Verification items for the finished model (mm, model axes). Face numbers are marked on the shaded views. A direction names the side the tool comes from. Give positions to 0.01 mm unless a question says otherwise; leave off trailing zeros. Loops run counter-clockwise (first coordinate to the right, second up) from the corner with the lowest first, then second, coordinate; pieces in that order, holes last. Notation, with made-up numbers: M 8.5,25 L 15.5,25 A16 ccw 15.5,34 Z; hole C -39.75,2.5 d4. An arc over 180 degrees is marked long. Use CSV: the item, a comma, the result in double quotes.
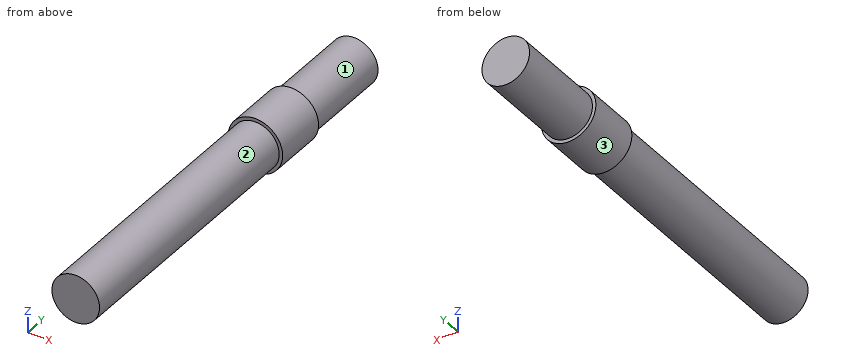
from build123d import *

# Parameters (mm, degrees)
F0_R      = 22.225
F1_DEPTH  = 406.4
F3_R      = 25.4
F4_DEPTH  = 50.8
F1_FACE_R = 22.225
F5_DEPTH  = 12.7


with BuildPart() as f1:
    # F0 (on Front) → F1 (new body)
    with BuildSketch(Plane.XZ):
        Circle(F0_R)
    extrude(amount=F1_DEPTH)

    # F3 (on offset) → F4 (join)
    with BuildSketch(Plane.XZ.offset(152.4)):
        Circle(F3_R)
    extrude(amount=-F4_DEPTH)

    # F1_face (on face) → F5 (cut)
    with BuildSketch(Plane(origin=(0, 0, 0), x_dir=(1, 0, 0), z_dir=(0, 1, 0))):
        Circle(F1_FACE_R)
    extrude(amount=-F5_DEPTH, mode=Mode.SUBTRACT)


solid = f1.part
(1) Depth check by flat-ended pin: pin 1 Ø4 at (y, z) = (-237.5, -2) entering from +X (3 decimals); pin 2 Ø1 at (x, y) = (-13.5, -360) entering from -Z; pin 3 Ø2 at (x, y) = (-11.5, -158) entering from +Z. Enter the tip coordinate at first touch or a pass-through.
Calculated:
pin 1,"stops at x = 22.225"
pin 2,"stops at z = -18.03"
pin 3,"stops at z = 19.59"
(2) Section check C-C on y = -169. Record the cut outline in (x, z) (3 decimals).
Calculated:
outline,"C 0,0 d44.45"
(3) Scan lines: L1, parallel to Y at x = 16.5, z = -17.5; L2, parallel to X at y = -370, z = 1.5; L3, parallel to Z at x = -19.5, y = -247. Record each from-to range of solid material in increasing order. Write a range as from..to.
Calculated:
L1,"y = -152.4..-101.6"
L2,"x = -22.17..22.17"
L3,"z = -10.66..10.66"
(4) Section check A-A on x = 0. Record the cut outline in (y, z) (3 decimals).
Calculated:
outline,"M -406.4,-22.225 L -152.4,-22.225 L -152.4,-25.4 L -101.6,-25.4 L -101.6,-22.225 L -12.7,-22.225 L -12.7,22.225 L -101.6,22.225 L -101.6,25.4 L -152.4,25.4 L -152.4,22.225 L -406.4,22.225 Z"
(5) Section check B-B on z = 0. Record the cut outline in (x, y) (3 decimals).
Calculated:
outline,"M -25.4,-152.4 L -22.225,-152.4 L -22.225,-406.4 L 22.225,-406.4 L 22.225,-152.4 L 25.4,-152.4 L 25.4,-101.6 L 22.225,-101.6 L 22.225,-12.7 L -22.225,-12.7 L -22.225,-101.6 L -25.4,-101.6 Z"
(6) Tool access check on the marked faces 1, 2 and 3. Record the directions out of +Z, -Z, +X, -X, +Y, -Y that give a thin tool (end or side, any length) a straight path to the whole face; none if there is none.
Calculated:
face 1,"+Y"
face 2,"-Y"
face 3,"+Y, -Y"
